```python
from build123d import *

# Parameters (mm, degrees)
SKETCH1_W             = 14.478
SKETCH1_H             = 22.225
BOSS_EXTRUDE1_DEPTH   = 7.493
F_0_80_TAPPED_HOLE1_D = 1.19126
F_2_CLEARANCE_HOLE1_D = 2.2606


with BuildPart() as part:
    # Sketch1 → Boss-Extrude1 (new body)
    with BuildSketch(Plane(origin=(0, 0, 0), x_dir=(1, 0, 0), z_dir=(0, 1, 0))):
        Rectangle(SKETCH1_W, SKETCH1_H)
    extrude(amount=BOSS_EXTRUDE1_DEPTH)

    # #0-80 Tapped Hole1 (through all)
    with Locations(Plane(origin=(0, 7.493, 0), x_dir=(-1, 0, 0), z_dir=(0, 1, 0))):
        with Locations((3, 9.525), (-3, 9.525)):
            Hole(F_0_80_TAPPED_HOLE1_D / 2)

    # #2 Clearance Hole1 (through all)
    with Locations(Plane(origin=(0, 7.493, 0), x_dir=(-1, 0, 0), z_dir=(0, 1, 0))):
        with Locations((5.6515, -9.525), (-5.6515, -9.525)):
            Hole(F_2_CLEARANCE_HOLE1_D / 2)


solid = part.part
```
Build history of the part. All positions in model axes, mm. Round coordinates to 2 decimals unless told otherwise and drop trailing zeros. Loops run counter-clockwise (first coordinate to the right, second up) from the corner with the lowest first, then second, coordinate; pieces in that order, holes last.
Item 1: Pin check, flat tips, straight feed: P1, Ø1.5, axis at x = -3, z = 9.525, coming from the +Y side; P2, Ø1.8, axis at x = 5.65, z = -9.52, coming from the +Y side. Stop position of each tip, or through.
Item 2: Two-plate mould, pull along Z, no slides. Class faces 1 (the face through (5.504, 3.694, -8.404)), 2 (the face through (0, 4, 11.112)), 3 (the face through (0, 7.493, 0)): released by +Z, released by -Z, zero draft, split by the parting line, or undercut.
Item 3: Saw through at C-C (y = 2.25). List the corners of the cut face in (x, z) (1 decimal).
Item 4: Saw through at B-B (z = -9.25). List the corners of the cut face in (x, y).
Item 5: Saw through at D-D (x = 5.25). List the corners of the cut face in (y, z).
Item 6: Drill centre lines: line 1 along Z through (x, y) = (-3, 5); line 2 along X through (y, z) = (5.5, -10); line 3 along X through (y, z) = (0.5, 9.75). Where is each one in solid material? Low to high.
Item 7: Saw through at A-A (x = -3). List the corners of the cut face in (y, z), then the cut area to 3 significant figures.
Worked answers:
1. P1: stops at y = 7.49
1. P2: passes through
2. face 1: undercut
2. face 2: released by +Z
2. face 3: zero draft
3. outline: (-7.2, -11.1) - (7.2, -11.1) - (7.2, 11.1) - (-7.2, 11.1) - close; hole circle Ø2.3 at (-5.7, -9.5); hole circle Ø1.2 at (-3, 9.5); hole circle Ø1.2 at (3, 9.5); hole circle Ø2.3 at (5.7, -9.5)
4. outline: (-7.24, 0) - (-6.75, 0) - (-6.75, 7.49) - (-7.24, 7.49) - close; (-4.56, 0) - (4.56, 0) - (4.56, 7.49) - (-4.56, 7.49) - close; (6.75, 0) - (7.24, 0) - (7.24, 7.49) - (6.75, 7.49) - close
5. outline: (0, -11.11) - (7.49, -11.11) - (7.49, -10.58) - (0, -10.58) - close; (0, -8.47) - (7.49, -8.47) - (7.49, 11.11) - (0, 11.11) - close
6. line 1: z = -11.11 to 8.93, 10.12 to 11.11
6. line 2: x = -7.24 to -6.68, -4.63 to 4.63, 6.68 to 7.24
6. line 3: x = -7.24 to -3.55, -2.45 to 2.45, 3.55 to 7.24
7. outline: (0, -11.11) - (7.49, -11.11) - (7.49, 8.93) - (0, 8.93) - close; (0, 10.12) - (7.49, 10.12) - (7.49, 11.11) - (0, 11.11) - close
7. area: 158 mm2
